Autodesk Inventor part; units mm, degrees
ref_plane "YZ Plane" through (0, 0, 0) normal (1, 0, 0) x (0, 1, 0)
ref_plane "XZ Plane" through (0, 0, 0) normal (0, 1, 0) x (-1, 0, 0)
ref_plane "XY Plane" through (0, 0, 0) normal (0, 0, 1) x (1, 0, 0)
sketch "Skizze1" plane through (0, 0, 0) normal (1, 0, 0) x (0, 1, 0)
  circle A0 centre (0, 0) radius 75
  dimension "d0" = 150
extrude "Extrusion1" add sketch "Skizze1" along normal blind 150
shell "Wandung1" thickness 10 removed faces 1 at (150, 17.7208, 28.0232)
chamfer "Fase1" distance 7 distance2 90 1 edges at (150, -65, 0) measured on face at (150, -32.1985, -63.7899)
chamfer "Fase2" distance 7 distance2 90 1 edges at (0, -75, 0) measured on face at (0, 17.7208, 28.0232)
properties part number "Blumentopf"
For this review, take the finished solid that the model builds, in its own axes (mm). A direction names the side the tool comes from. Coordinates: 2 decimals unless noted, no trailing zeros. Write each loop counter-clockwise with the first axis right and the second up, starting at its lowest first coordinate (ties: lowest second). Pieces come first, ordered by that corner, then holes. Notation, with made-up numbers: (-10.75, 17) -> (-6.75, 17) arc R26 ccw to (-6.75, 56) -> close; hole circle Ø11 at (12.5, 31). An arc over 180 degrees is marked (long way). Write each question's results on one line, items separated by ' | '. Start each with the question number.
1) Consider section A-A (z = 0). Write out the cut boundary in (x, y).
2) For faces 1 (the face through (34.65, 62, -19.52)), 2 (the face through (35.63, -15.34, -69.09)), list the 3-axis set-ups (+Z, -Z, +X, -X, +Y, -Y) from which the entire face can be reached by the end or side of a thin tool; tool diameter is ignored.
3) Consider section D-D (x = 96). Write out the cut boundary in (y, z), plus the area to 3 significant figures.
4) Wall thickness on L1, parallel to X at y = 15.5, z = -27.5; L2, parallel to Y at x = 60, z = 14.5; L3, parallel to Y at x = 74, z = 53.5: over which ranges is each line inside the solid? List them lowest first. Write a range as [from, to].
5) Insertion check: pin 1 (1 mm diameter, centred on y = 22.5, z = -51, fed in from +X); pin 2 (8 mm diameter, centred on x = 38, z = -40.5, fed in from +Y); pin 3 (6 mm diameter, centred on x = 21.5, y = -55.5, fed in from +Z). Each pin has a flat end and moves straight along its axis. Give the tip position at first contact, or say it passes through.
6) Consider section C-C (x = 13.5). Write out the cut boundary in (y, z).
7) The part is to be moulded in two halves that separate along Y. For faces 3 (the face through (150, -67, 28)), 4 (the face through (95.63, 64.64, 20.36)), 5 (the face through (119.58, -9.764, -74.362)), 6 (the face through (10, -1, 1)), say which applies: +Y half, -Y half, draft (parallel to the pull), parting line (faces both ways), or undercut.
Geometry says:
1) outline: (0, -68) -> (90, -75) -> (150, -75) -> (150, -72) -> (60, -65) -> (10, -65) -> (10, 65) -> (60, 65) -> (150, 72) -> (150, 75) -> (90, 75) -> (0, 68) -> close
2) face 1: +X | face 2: -X
3) outline: circle Ø150 at (0, 0); hole circle Ø135.6 at (0, 0) | area: 3,230 mm^2
4) L1: [0, 10] | L2: [-71.21, -63.36], [63.36, 71.21] | L3: [-50.77, -38.8], [38.8, 50.77]
5) pin 1: x = 10 | pin 2: y = 60.87 | pin 3: z = 45.82
6) outline: circle Ø138.1 at (0, 0); hole circle Ø130 at (0, 0)
7) face 3: draft | face 4: undercut | face 5: parting line | face 6: undercut
